For this review, take the finished solid that the model builds, in its own axes (mm). Give positions to 0.01 mm unless a question says otherwise; leave off trailing zeros. Order: outer loops, then holes, each group sorted by start corner. A loop starts at its lowest first (then second) coordinate and runs counter-clockwise, first axis right, second up.
from build123d import *

# Parameters (mm, degrees)
SKETCH1_W           = 320
SKETCH1_H           = 320
SKETCH1_R           = 1.65
SKETCH1_R_2         = 1.35
SKETCH1_R_3         = 2.25
SKETCH1_R_4         = 15
BOSS_EXTRUDE1_DEPTH = 3
FILLET1_R           = 10


with BuildPart() as part:
    # Sketch1 → Boss-Extrude1 (new body)
    with BuildSketch(Plane(origin=(0, 0, 0), x_dir=(1, 0, 0), z_dir=(0, 1, 0))):
        with Locations((45.2, -56.43)):
            Rectangle(SKETCH1_W, SKETCH1_H)
        with Locations((101.6, 16)):
            Circle(SKETCH1_R, mode=Mode.SUBTRACT)
        with Locations((2.15, 2.15)):
            Circle(SKETCH1_R, mode=Mode.SUBTRACT)
        with Locations((33.15, 2.15)):
            Circle(SKETCH1_R, mode=Mode.SUBTRACT)
        with Locations((2.15, 53.15)):
            Circle(SKETCH1_R, mode=Mode.SUBTRACT)
        with Locations((57.1, 76.14)):
            Circle(SKETCH1_R, mode=Mode.SUBTRACT)
        with Locations((163.7, 2.57)):
            Circle(SKETCH1_R_2, mode=Mode.SUBTRACT)
        with Locations((114.7, 2.57)):
            Circle(SKETCH1_R_2, mode=Mode.SUBTRACT)
        with Locations((163.7, 60.57)):
            Circle(SKETCH1_R_2, mode=Mode.SUBTRACT)
        with Locations((114.7, 60.57)):
            Circle(SKETCH1_R_2, mode=Mode.SUBTRACT)
        with Locations((-14.3, -8.93)):
            Circle(SKETCH1_R, mode=Mode.SUBTRACT)
        with Locations((-66.8, -8.93)):
            Circle(SKETCH1_R, mode=Mode.SUBTRACT)
        with Locations((-14.3, 92.07)):
            Circle(SKETCH1_R, mode=Mode.SUBTRACT)
        with Locations((-66.8, 92.07)):
            Circle(SKETCH1_R, mode=Mode.SUBTRACT)
        with Locations((-35.3, -85.43)):
            Circle(SKETCH1_R_3, mode=Mode.SUBTRACT)
        with Locations((125.7, -85.43)):
            Circle(SKETCH1_R_3, mode=Mode.SUBTRACT)
        with Locations((125.7, -185.43)):
            Circle(SKETCH1_R_3, mode=Mode.SUBTRACT)
        with Locations((-35.3, -185.43)):
            Circle(SKETCH1_R_3, mode=Mode.SUBTRACT)
        with Locations((45.2, -135.43)):
            Circle(SKETCH1_R_4, mode=Mode.SUBTRACT)
    extrude(amount=BOSS_EXTRUDE1_DEPTH)

    # Fillet1
    fillet1_edges = [part.edges().sort_by_distance(p)[0] for p in [
        (205.2, 1.5, 216.43),
        (-114.8, 1.5, 216.43),
        (-114.8, 1.5, -103.57),
        (205.2, 1.5, -103.57),
    ]]
    fillet(fillet1_edges, radius=FILLET1_R)


solid = part.part
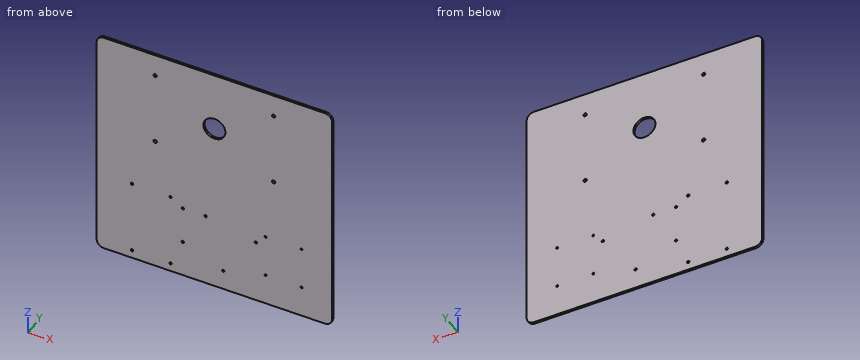
1) We need section A-A on z = 135.43. Give the boundary of the cut face in (x, y).
Answer sheet:
outline: (-114.8, 0) - (30.2, 0) - (30.2, 3) - (-114.8, 3) - close; (60.2, 0) - (205.2, 0) - (205.2, 3) - (60.2, 3) - close
2) We need section B-B on x = 45.2. Give the boundary of the cut face in (y, z).
Answer sheet:
outline: (0, -103.57) - (3, -103.57) - (3, 120.43) - (0, 120.43) - close; (0, 150.43) - (3, 150.43) - (3, 216.43) - (0, 216.43) - close
3) To check wall thickness, follow line 1 (Z direction, x = -14.3, y = 1.2); line 2 (Z direction, x = 114.7, y = 0.85); line 3 (X direction, y = 1.65, z = -76.14). State the ranges of each line that lie inside material, in increasing order.
Answer sheet:
line 1: z = -103.57 to -93.72, -90.42 to 7.28, 10.58 to 216.43
line 2: z = -103.57 to -61.92, -59.22 to -3.92, -1.22 to 216.43
line 3: x = -114.8 to 55.45, 58.75 to 205.2
4) Clearance check with a flat-ended pin moving along its axis: pin 1 (5.5 mm diameter, centred on x = -14.3, z = -92.07, fed in from -Y). State where the tip first meets the part, or that it passes through.
Answer sheet:
pin 1: stops at y = 0
